Verification items for the finished model (mm, model axes). Face numbers are marked on the shaded views. A direction names the side the tool comes from. Round coordinates to 2 decimals unless told otherwise and drop trailing zeros. Write each loop counter-clockwise with the first axis right and the second up, starting at its lowest first coordinate (ties: lowest second). Pieces come first, ordered by that corner, then holes. Notation, with made-up numbers: M 27,44.25 L 71,44.25 A26 ccw 71,63.25 Z; hole C 24,3.25 d11. An arc over 180 degrees is marked long. Write each question's results on one line, items separated by ' | '.
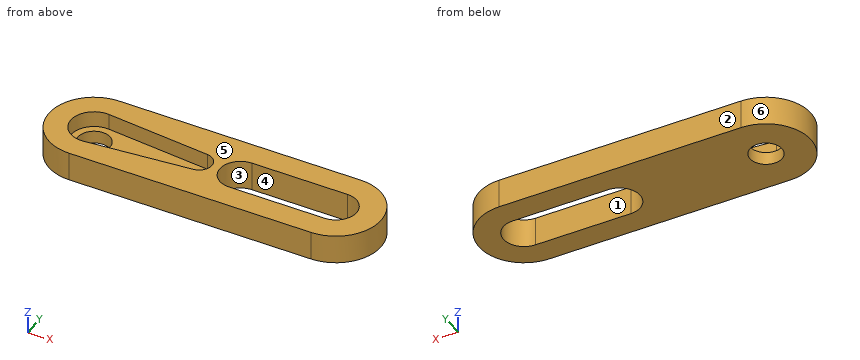
from build123d import *

# Parameters (mm, degrees)
MAIN_DEPTH            = 2.5
ESQUISSE2_R           = 2.5
ORIGINALBRACKET_DEPTH = 2
CUT_EXTRUDE1_DEPTH    = 3


with BuildPart() as part:
    # Esquisse1 → Main (new body)
    with BuildSketch(Plane.XY):
        with BuildLine():
            Line((0, 7), (38, 7))
            ThreePointArc((38, 7), (45, 0), (38, -7))
            Line((38, -7), (0, -7))
            ThreePointArc((0, -7), (-7, 0), (0, 7))
        make_face()
        with BuildLine():
            Line((0.349090909, 3.583034404), (16.693939394, 1.990574669))
            ThreePointArc((16.693939394, 1.990574669), (18.5, 0), (16.693939394, -1.990574669))
            Line((16.693939394, -1.990574669), (0.349090909, -3.583034404))
            ThreePointArc((0.349090909, -3.583034404), (-3.6, 0), (0.349090909, 3.583034404))
        make_face(mode=Mode.SUBTRACT)
        with BuildLine():
            Line((23, 3.2), (38, 3.2))
            ThreePointArc((38, 3.2), (41.2, 0), (38, -3.2))
            Line((38, -3.2), (23, -3.2))
            ThreePointArc((23, -3.2), (19.8, 0), (23, 3.2))
        make_face(mode=Mode.SUBTRACT)
    extrude(amount=MAIN_DEPTH)

    # Esquisse2 → OriginalBracket (add)
    with BuildSketch(Plane(origin=(0, 0, 0), x_dir=(-1, 0, 0), z_dir=(0, 0, -1))):
        with BuildLine():
            Line((0, -7), (-38, -7))
            ThreePointArc((-38, -7), (-45, 0), (-38, 7))
            Line((-38, 7), (0, 7))
            ThreePointArc((0, 7), (7, 0), (0, -7))
        make_face()
        Circle(ESQUISSE2_R, mode=Mode.SUBTRACT)
    extrude(amount=ORIGINALBRACKET_DEPTH)

    # Sketch1 → Cut-Extrude1 (cut, through all)
    with BuildSketch(Plane.XY):
        with BuildLine():
            Line((23, 3.2), (38, 3.2))
            ThreePointArc((38, 3.2), (41.2, 0), (38, -3.2))
            Line((38, -3.2), (23, -3.2))
            ThreePointArc((23, -3.2), (19.8, 0), (23, 3.2))
        make_face()
    extrude(amount=-CUT_EXTRUDE1_DEPTH, mode=Mode.SUBTRACT)


solid = part.part
1) Sectioned sample at C-C, the plane x = 2. Record the cut outline in (y, z).
Calculated:
outline: M -7,-2 L -1.5,-2 L -1.5,0 L -3.42,0 L -3.42,2.5 L -7,2.5 Z; M 1.5,-2 L 7,-2 L 7,2.5 L 3.42,2.5 L 3.42,0 L 1.5,0 Z
2) Draft check along X on the marked faces 3, 4, 5 and 6. Enter one of: pulls with the +X half, pulls with the -X half, needs draft (parallel to the pull), parting line crosses it, or undercut.
Calculated:
face 3: undercut | face 4: undercut | face 5: needs draft | face 6: pulls with the -X half
3) Sectioned sample at D-D, the plane x = 13.5. Record the cut outline in (y, z), and give its area (3 significant figures).
Calculated:
outline: M -7,-2 L 7,-2 L 7,2.5 L 2.3,2.5 L 2.3,0 L -2.3,0 L -2.3,2.5 L -7,2.5 Z | area: 51.5 mm²
4) Depth check by flat-ended pin: P1, Ø2, axis at x = 9.5, y = 0.5, coming from the +Z side; P2, Ø2, axis at x = 31, y = -1, coming from the +Z side. Enter the tip coordinate at first touch or a pass-through.
Calculated:
P1: stops at z = 0 | P2: passes through
5) Sectioned sample at A-A, the plane y = 0. Record the cut outline in (x, z), and give its area (4 significant figures).
Calculated:
outline: M -7,-2 L -2.5,-2 L -2.5,0 L -3.6,0 L -3.6,2.5 L -7,2.5 Z; M 2.5,-2 L 19.8,-2 L 19.8,2.5 L 18.5,2.5 L 18.5,0 L 2.5,0 Z; M 41.2,-2 L 45,-2 L 45,2.5 L 41.2,2.5 Z | area: 72.45 mm²
6) Sectioned sample at B-B, the plane z = -0.5. Record the cut outline in (x, y).
Calculated:
outline: M 0,-7 L 38,-7 A7 ccw 38,7 L 0,7 A7 ccw Z; hole C 0,0 d5; hole M 23,-3.2 L 38,-3.2 A3.2 ccw 38,3.2 L 23,3.2 A3.2 ccw Z
7) Material ranges on line 1 (X direction, y = 1.25, z = 2.3); line 2 (Y direction, x = 0, z = 1.95); line 3 (Y direction, x = 29, z = 0.1), recorded low to high. Write a range as [from, to].
Calculated:
line 1: x = [-6.89, -3.38], [18.06, 20.05], [40.95, 44.89] | line 2: y = [-7, -3.6], [3.6, 7] | line 3: y = [-7, -3.2], [3.2, 7]
8) Access from +Z, -Z, +X, -X, +Y, -Y to the whole of each face (thin tool, end or side, straight path). Record for the marked faces 1 and 2.
Calculated:
face 1: +Z, -Z | face 2: +Z, -Z, +X, -X, +Y
